Could you check a few things on this model? Use its own coordinates, in mm. A direction names the side the tool comes from. Give positions to 0.01 mm unless a question says otherwise; leave off trailing zeros. Write each loop counter-clockwise with the first axis right and the second up, starting at its lowest first coordinate (ties: lowest second). Pieces come first, ordered by that corner, then holes. Notation, with made-up numbers: (65.25, 43) - (88.25, 43) arc R19 ccw to (88.25, 65) - close; hole circle Ø6 at (17.25, 74). An arc over 180 degrees is marked (long way). Use one line per item in the form item = value.
```python
from build123d import *

# Parameters (mm, degrees)
PAD168_DEPTH              = 22
SKETCH247_W               = 4
SKETCH247_H               = 4
PAD167_DEPTH              = 13.5
SKETCH244_R               = 0.45
SKETCH244_W               = 0.8
SKETCH244_H               = 9.5
POCKET031_DEPTH           = 5
BODY041_PLACEMENT_ANGLE   = 90
FUSION004_PLACEMENT_ANGLE = 29


with BuildPart() as segment_wing004:
    # Sketch240 → Pad168 (new body)
    with BuildSketch(Plane.XY):
        with BuildLine():
            ThreePointArc((1.377124, 11.215772), (-3.957343, 10.584396), (-8.397537, 7.561176))
            Line((-8.397537, 7.561176), (-8.917738, 8.029567))
            ThreePointArc((1.462432, 11.910554), (-4.202489, 11.240066), (-8.917738, 8.029567))
            Line((1.377124, 11.215772), (1.462432, 11.910554))
        make_face()
    extrude(amount=PAD168_DEPTH)


with BuildPart() as segment_wing004_1:
    # Body044 placement: moved
    add(segment_wing004.part.moved(Location((0, 0, -9))))


with BuildPart() as segment_on004:
    # Sketch247 → Pad167 (new body)
    with BuildSketch(Plane.XY):
        with Locations((0, 6)):
            Rectangle(SKETCH247_W, SKETCH247_H)
    extrude(amount=PAD167_DEPTH)

    # Sketch244 (on Face1 of Pad167) → Pocket031 (cut)
    with BuildSketch(Plane(origin=(0, 8, 0), x_dir=(-1, 0, 0), z_dir=(0, 1, 0))):
        with Locations((0, 11.5)):
            Circle(SKETCH244_R)
        with Locations((-1.6, 4.75)):
            Rectangle(SKETCH244_W, SKETCH244_H)
        with Locations((1.6, 4.75)):
            Rectangle(SKETCH244_W, SKETCH244_H)
    extrude(amount=-POCKET031_DEPTH, mode=Mode.SUBTRACT)


with BuildPart() as segment_on004_1:
    # Body041 placement: moved
    add(segment_on004.part.moved(Location((0, 11.5, 2))).rotate(Axis((0, 11.5, 2), (1, 0, 0)), BODY041_PLACEMENT_ANGLE))

    # Fusion004: union Segment_Wing004
    add(segment_wing004_1.part)


with BuildPart() as segment_on004_2:
    # Fusion004 placement: moved
    add(segment_on004_1.part.rotate(Axis((0, 0, 0), (0, 0, -1)), FUSION004_PLACEMENT_ANGLE))


solid = segment_on004_2.part
```
1. If we mould it in two halves opening along Y, with no side actions, what happens to faces 3 (the face through (1.6, 11.4, 13)), 4 (the face through (1.76, -0.95, 7.97)), 5 (the face through (1.853, 11.856, 1.846)), 6 (the face through (2.19, 6.43, 8.03))? For each: pulls with the +Y half, pulls with the -Y half, needs draft (parallel to the pull), parting line crosses it, or undercut.
Response values:
face_3 = needs draft
face_4 = pulls with the -Y half
face_5 = pulls with the +Y half
face_6 = undercut
2. Imagine slicing it at D-D, the plane y = 5.5. List the corners of the cut face in (x, z) for me, and give its area (3 significant figures).
Response values:
outline = (1.68, 6) - (4.42, 6) - (4.42, 10) - (1.68, 10) - close
area = 11.0 mm²
3. For pin 1 (3 mm diameter, centred on x = 1.5, z = 5, fed in from +Y); pin 2 (4.5 mm diameter, centred on x = 2.5, y = 2.5, fed in from +Z); pin 3 (4 mm diameter, centred on y = 6, z = 4.5, fed in from +X); pin 4 (1.5 mm diameter, centred on x = -2, z = -1, fed in from -Y), each with a flat end and sliding along its axis, tell me the tip position at first contact or that it passes through.
Response values:
pin_1 = 12
pin_2 = 10
pin_3 = 5.43
pin_4 = 10.96
4. Which directions (+Z, -Z, +X, -X, +Y, -Y) give clear straight access to the entire face, cutting with the end or side of a thin tool? Please do faces 1 (the face through (-1.74, 0.99, 7.97)), 2 (the face through (1.6, 11.4, -9)).
Response values:
face_1 = +Z, -Z, -X
face_2 = -Z, +X, -X, +Y, -Y
5. If I drill on line 1 (Y direction, x = 0, z = 8.25); line 2 (Y direction, x = 3.5, z = 6.75); line 3 (Y direction, x = 0, z = 2), over which ranges is the centre line in solid material (lowest first)? Write a range as from..to.
Response values:
line_1 = -2.29..-0.45, 0.45..2.48, 11.3..12
line_2 = 3.84..8.79, 10.74..11.48
line_3 = 11.3..12
6. Imagine slicing it at A-A, the plane x = 2.25. List the corners of the cut face in (y, z) for me.
Response values:
outline = (-0.07, 6) - (1.04, 6) - (1.04, 10) - (-0.07, 10) - close; (1.58, 6) - (6.53, 6) - (6.53, 10) - (1.58, 10) - close; (11.07, -9) - (11.79, -9) - (11.79, 13) - (11.07, 13) - close
7. Imagine slicing it at B-B, the plane z = 2.75. List the corners of the cut face in (x, y) for me.
Response values:
outline = (-3.91, 11.35) - (-3.68, 10.68) arc R11.3 cw to (6.64, 9.14) - (7.05, 9.71) arc R12 ccw to start
8. Imagine slicing it at C-C, the plane x = 6. List the corners of the cut face in (y, z) for me, and give its area (3 significant figures).
Response values:
outline = (8.35, 6) - (9.58, 6) - (9.58, -9) - (10.39, -9) - (10.39, 13) - (9.58, 13) - (9.58, 10) - (8.35, 10) - close
area = 22.9 mm²
